Here's how the part is built. I have some questions about the finished solid (model axes, mm). A direction names the side the tool comes from. Round coordinates to 2 decimals unless told otherwise and drop trailing zeros. Write each loop counter-clockwise with the first axis right and the second up, starting at its lowest first coordinate (ties: lowest second). Pieces come first, ordered by that corner, then holes. Notation, with made-up numbers: (51.25, 61.5) - (87.25, 61.5) arc R31 cw to (87.25, 94.5) - close; hole circle Ø4 at (81.5, -7.5). An arc over 180 degrees is marked (long way). One line per item, written item: value. Start each with the question number.
Item 1: If I drill on line 1 (X direction, y = -90, z = 0.9); line 2 (X direction, y = 98.5, z = 2.7); line 3 (Y direction, x = -61, z = 3) (3 decimals), over which ranges is the centre line in solid material (lowest first)?
Item 2: Imagine slicing it at D-D, the plane z = 1.8. Count the separate pieces of the cut face and the enclosed holes in it, then the cut area to 3 significant figures.
Item 3: Imagine slicing it at C-C, the plane y = 49.5. Please give me the cut outline in (x, z), then the cut area to 3 significant figures.
Item 4: Thinking about a two-plate mould opening in X: for faces 3 (the face through (126.96, 1, 3)), 4 (the face through (37.919, -92, 3)), 5 (the face through (2, 2, 0)), which applies, released by +X, released by -X, zero draft, split by the parting line, or undercut?
Item 5: For faces 1 (the face through (-37.919, -92, 3)), 2 (the face through (2, 2, 5.334)), which set-ups out of +Z, -Z, +X, -X, +Y, -Y let a thin tool reach every point of the face, with its end or its side?
Item 6: Imagine slicing it at A-A, the plane y = 90. Please give me the cut outline in (x, z), then the cut area to 3 significant figures.
Item 7: For P1, Ø3, axis at x = -96, z = 4, coming from the +Y side; P2, Ø2.5, axis at x = -34, z = 2, coming from the -Y side; P3, Ø2.5, axis at x = -61, z = 2, coming from the +Y side; P4, Ø1.6, axis at x = -74.54, y = 74.54, coming from the +Z side, each with a flat end and sliding along its axis, tell me the tip position at first contact or that it passes through.
Item 8: Imagine slicing it at B-B, the plane x = 82. Please give me the cut outline in (y, z).
```python
from build123d import *

# Parameters (mm, degrees)
SKETCH1_W                     = 5.334
SKETCH1_H                     = 46.99
BASE_PLATFORM_DEPTH           = 5.334
SKETCH5_R                     = 0.889
PERIMETER_STACKING_CUTS_DEPTH = 5.334
SKETCH6_W                     = 5.334
SKETCH6_H                     = 19.05
SKID_HOLES_DEPTH              = 5.334


with BuildPart() as part:
    # Sketch1 → Base Platform (new body)
    with BuildSketch(Plane.XY):
        with BuildLine():
            Line((126.959765957, -36.195), (108.417765957, -36.195))
            ThreePointArc((108.417765957, -36.195), (0, -114.3), (-108.417765957, -36.195))
            Line((-108.417765957, -36.195), (-126.959765957, -36.195))
            Line((-126.959765957, -36.195), (-126.959765957, 36.195))
            Line((-126.959765957, 36.195), (-108.417765957, 36.195))
            ThreePointArc((-108.417765957, 36.195), (0, 114.3), (108.417765957, 36.195))
            Line((108.417765957, 36.195), (126.959765957, 36.195))
            Line((126.959765957, 36.195), (126.959765957, -36.195))
        make_face()
        with Locations((-116.418765957, 0)):
            Rectangle(SKETCH1_W, SKETCH1_H, mode=Mode.SUBTRACT)
        with Locations((62.062765957, 0)):
            Rectangle(SKETCH1_W, SKETCH1_H, mode=Mode.SUBTRACT)
        with Locations((-62.062765957, 0)):
            Rectangle(SKETCH1_W, SKETCH1_H, mode=Mode.SUBTRACT)
        with Locations((116.418765957, 0)):
            Rectangle(SKETCH1_W, SKETCH1_H, mode=Mode.SUBTRACT)
    extrude(amount=BASE_PLATFORM_DEPTH)

    # Sketch5 → Perimeter stacking cuts (cut)
    with BuildSketch(Plane(origin=(0, 0, 0), x_dir=(-1, 0, 0), z_dir=(0, 0, -1))):
        with Locations((0, 105.41)):
            Circle(SKETCH5_R)
        with Locations((0, -105.41)):
            Circle(SKETCH5_R)
        with Locations((-74.536125805, 74.536125805)):
            Circle(SKETCH5_R)
        with Locations((74.536125805, 74.536125805)):
            Circle(SKETCH5_R)
        with Locations((74.536125805, -74.536125805)):
            Circle(SKETCH5_R)
        with Locations((-74.536125805, -74.536125805)):
            Circle(SKETCH5_R)
    extrude(amount=-PERIMETER_STACKING_CUTS_DEPTH, mode=Mode.SUBTRACT)

    # Sketch6 → Skid Holes (cut)
    with BuildSketch(Plane(origin=(0, 0, 0), x_dir=(-1, 0, 0), z_dir=(0, 0, -1))):
        with Locations((-35.251559841, 92.105443783)):
            Rectangle(SKETCH6_W, SKETCH6_H)
        with Locations((35.251559841, 92.105443783)):
            Rectangle(SKETCH6_W, SKETCH6_H)
        with Locations((35.251559841, -92.105443783)):
            Rectangle(SKETCH6_W, SKETCH6_H)
        with Locations((-35.251559841, -92.105443783)):
            Rectangle(SKETCH6_W, SKETCH6_H)
    extrude(amount=-SKID_HOLES_DEPTH, mode=Mode.SUBTRACT)


solid = part.part
```
Values follow:
1. line 1: x = -70.46 to -37.92, -32.58 to 32.58, 37.92 to 70.46
1. line 2: x = -57.98 to -37.92, -32.58 to 32.58, 37.92 to 57.98
1. line 3: y = -96.662 to -23.495, 23.495 to 96.662
2. separate pieces: 1
2. enclosed holes: 14
2. area: 41,700 mm^2
3. outline: (-103.03, 0) - (103.03, 0) - (103.03, 5.33) - (-103.03, 5.33) - close
3. area: 1,100 mm^2
4. face 3: released by +X
4. face 4: undercut
4. face 5: zero draft
5. face 1: +Z, -Z
5. face 2: +Z, +X, -X, +Y, -Y
6. outline: (-70.46, 0) - (-37.92, 0) - (-37.92, 5.33) - (-70.46, 5.33) - close; (-32.58, 0) - (32.58, 0) - (32.58, 5.33) - (-32.58, 5.33) - close; (37.92, 0) - (70.46, 0) - (70.46, 5.33) - (37.92, 5.33) - close
6. area: 695 mm^2
7. P1: stops at y = 64.3
7. P2: stops at y = -109.51
7. P3: stops at y = 97.44
7. P4: passes through
8. outline: (-79.63, 0) - (79.63, 0) - (79.63, 5.33) - (-79.63, 5.33) - close
